Study the drawing (mm; zero at the part's minimum x, y, z) and answer. A direction names the side the tool comes from. Round coordinates to 2 decimals unless told otherwise and drop trailing zeros. Loops run counter-clockwise (first coordinate to the right, second up) from the corner with the lowest first, then second, coordinate; pieces in that order, holes last. Notation, with made-up numbers: (16, -2) - (20, -2) arc R18 cw to (20, 14) - close; hole circle Ø5 at (71.25, 21). An arc over 180 degrees is marked (long way). One line per item, written item: value.
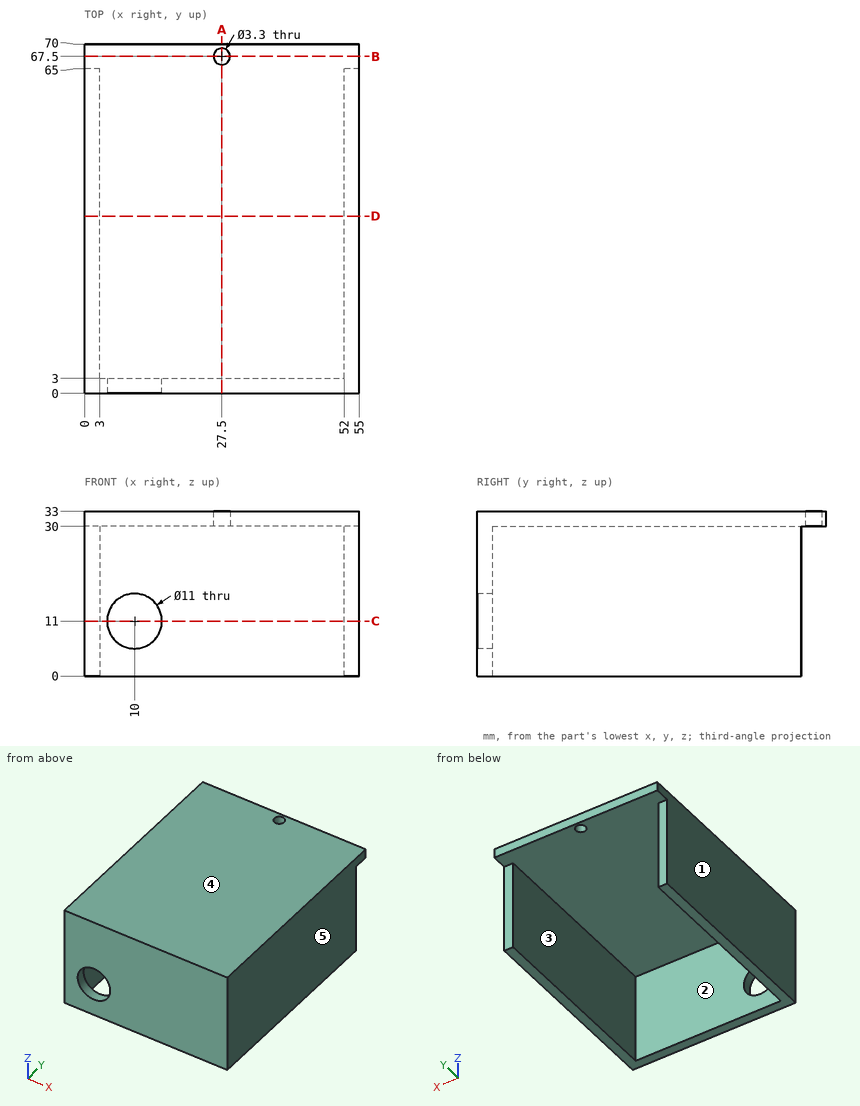
1) A cutting plane is placed at D-D on y = 35.5. Give the vertices of the cut face in (x, z).
Final values:
outline: (0, 0) - (3, 0) - (3, 30) - (52, 30) - (52, 0) - (55, 0) - (55, 33) - (0, 33) - close
2) For a pull along X with two mould halves and no side action, classify the marked faces 3, 4 and 5 as released by +X, released by -X, zero draft, split by the parting line, or undercut.
Final values:
face 3: undercut
face 4: zero draft
face 5: released by +X
3) A cutting plane is placed at C-C on z = 11. Give the vertices of the cut face in (x, y), and give its area (3 significant figures).
Final values:
outline: (0, 0) - (4.5, 0) - (4.5, 3) - (3, 3) - (3, 65) - (0, 65) - close; (15.5, 0) - (55, 0) - (55, 65) - (52, 65) - (52, 3) - (15.5, 3) - close
area: 504 mm2
4) Consider L1, parallel to Y at x = 27.5, z = 31.15; L2, parallel to X at y = 52.5, z = 10; L3, parallel to Z at x = 10, y = 2. Determine where each line is inside the solid, lowest interval first.
Final values:
L1: 0 to 65.85, 69.15 to 70
L2: 0 to 3, 52 to 55
L3: 0 to 5.5, 16.5 to 33
5) A cutting plane is placed at A-A on x = 27.5. Give the vertices of the cut face in (y, z), and give its area (3 significant figures).
Final values:
outline: (0, 0) - (3, 0) - (3, 30) - (65.85, 30) - (65.85, 33) - (0, 33) - close; (69.15, 30) - (70, 30) - (70, 33) - (69.15, 33) - close
area: 290 mm2
6) For the marked faces 1 and 2, determine the directions among +Z, -Z, +X, -X, +Y, -Y from which every point of the face is accessible in a straight line to the end or side of a thin tool.
Final values:
face 1: +Z, -Z, -X, +Y, -Y
face 2: -Z, +Y
7) Each of these flat-tipped pins is pushed along its axis until it touches: pin 1 Ø15 at (x, z) = (37.5, 14.5) entering from +Y; pin 2 Ø2.5 at (x, z) = (53, 11) entering from +Y; pin 3 Ø2 at (x, y) = (49, 39.5) entering from -Z. Where does it stop, or does it pass through?
Final values:
pin 1: y = 3
pin 2: y = 65
pin 3: z = 30
8) A cutting plane is placed at B-B on y = 67.5. Give the vertices of the cut face in (x, z), and give its area (3 significant figures).
Final values:
outline: (0, 30) - (25.85, 30) - (25.85, 33) - (0, 33) - close; (29.15, 30) - (55, 30) - (55, 33) - (29.15, 33) - close
area: 155 mm2
